Read the model definition and answer for the solid it produces. Units are mm, in the model's axes. Face numbers are marked on the shaded views. A direction names the side the tool comes from. Coordinates: 2 decimals unless noted, no trailing zeros. Order: outer loops, then holes, each group sorted by start corner. A loop starts at its lowest first (then second) coordinate and runs counter-clockwise, first axis right, second up. Notation, with made-up numbers: M -6,-34.5 L 7,-34.5 A28 cw 7,-8.5 Z; hole C -7,-29 d8. An arc over 180 degrees is marked long. Put each result on its own line as item: value.
from build123d import *

# Parameters (mm, degrees)
CUT_EXTRUDE1_DEPTH  = 5
CUT_EXTRUDE12_DEPTH = 5.5
CHAMFER1_SIZE       = 2


with BuildPart() as part:
    # Sketch1 → Revolve1 (revolve)
    with BuildSketch(Plane(origin=(0, 0, 0), x_dir=(1, 0, 0), z_dir=(0, 1, 0)), mode=Mode.PRIVATE) as revolve1_sk:
        Polygon((0, 0), (0, -400), (20, -400), (20, -310), (22.5, -310), (22.5, -220), (25, -220), (25, -140), (28, -140), (28, -130), (25, -130), (25, -30), (22.5, -30), (22.5, 0), align=None)
    revolve(revolve1_sk.sketch.rotate(Axis((0, 0, 0), (0, 0, 1)), 180), axis=Axis((0, 0, 0), (0, 0, 1)))

    # Sketch3 → Cut-Extrude1 (cut)
    with BuildSketch(Plane(origin=(0, 20, 400), x_dir=(0, 0, 1), z_dir=(0, -1, 0))):
        with BuildLine():
            Line((-25, 6), (-75, 6))
            ThreePointArc((-75, 6), (-81, 0), (-75, -6))
            Line((-75, -6), (-25, -6))
            ThreePointArc((-25, -6), (-19, 0), (-25, 6))
        make_face()
    extrude(amount=CUT_EXTRUDE1_DEPTH, mode=Mode.SUBTRACT)

    # Sketch32 → Cut-Extrude12 (cut)
    with BuildSketch(Plane(origin=(0, 25, 220), x_dir=(0, 0, 1), z_dir=(0, -1, 0))):
        with BuildLine():
            Line((-27, 7), (-67, 7))
            ThreePointArc((-67, 7), (-74, 0), (-67, -7))
            Line((-67, -7), (-27, -7))
            ThreePointArc((-27, -7), (-20, 0), (-27, 7))
        make_face()
    extrude(amount=CUT_EXTRUDE12_DEPTH, mode=Mode.SUBTRACT)

    # Chamfer1
    chamfer1_edges = [part.edges().sort_by_distance(p)[0] for p in [
        (20, 0, 400),
    ]]
    chamfer(chamfer1_edges, length=CHAMFER1_SIZE)


solid = part.part
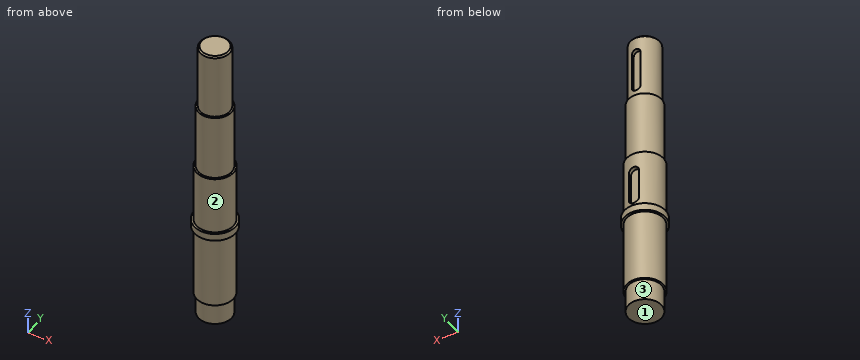
Q1. Given pin 1 (4 mm diameter, centred on x = -20, z = 54, fed in from -Y); pin 2 (1 mm diameter, centred on x = -14.5, z = 321.5, fed in from -Y); pin 3 (1.3 mm diameter, centred on y = 22, z = 182, fed in from +X), each flat-ended and moving along its own axis, determine where each tip first touches the part or whether it passes through.
Answers below:
pin 1: stops at y = -17.35
pin 2: stops at y = -14.28
pin 3: stops at x = 13.01
Q2. Find section C-C on z = 120. Write down the section's boundary in (x, y), plus the area to 3 significant figures.
Answers below:
outline: C 0,0 d50
area: 1,960 mm^2
Q3. A tool of negligible diameter and unlimited length cuts with its end or side. For the marked faces 1, 2 and 3, from which of +Z, -Z, +X, -X, +Y, -Y can it reach the whole face along a straight path? Write none if from no direction.
Answers below:
face 1: -Z, +X, -X, +Y, -Y
face 2: +Z
face 3: -Z
Q4. Find section D-D on z = 300. Write down the section's boundary in (x, y), plus the area to 3 significant figures.
Answers below:
outline: C 0,0 d45
area: 1,590 mm^2
Q5. Find section B-B on z = 187.5. Write down the section's boundary in (x, y), plus the area to 3 significant figures.
Answers below:
outline: M -7,19.5 L -7,24 A25 ccw long 7,24 L 7,19.5 Z
area: 1,890 mm^2
Q6. Consider line 1 along Z through (x, y) = (22.5, 5); line 2 along Z through (x, y) = (19.5, -7.5); line 3 along Y through (x, z) = (2, 83.5). Determine where each line is inside the solid, lowest interval first.
Answers below:
line 1: z = 30 to 220
line 2: z = 0 to 310
line 3: y = -24.92 to 24.92
